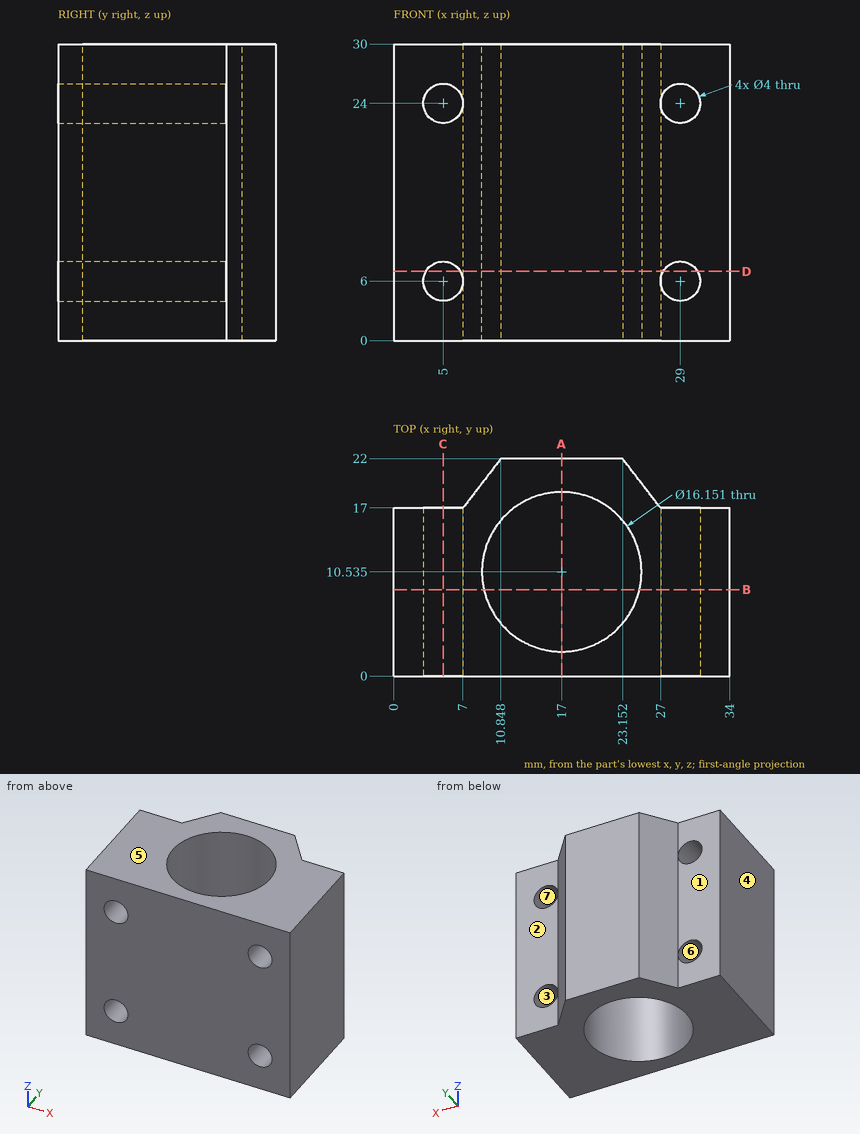
Study the drawing (mm; zero at the part's minimum x, y, z) and answer. A direction names the side the tool comes from. Give positions to 0.01 mm unless a question says otherwise; leave off trailing zeros. Write each loop counter-clockwise with the first axis right and the second up, starting at its lowest first coordinate (ties: lowest second). Pieces come first, ordered by that corner, then holes. Notation, with made-up numbers: (71.25, -32.75) - (75.25, -32.75) arc R24 cw to (75.25, -19.75) - close; hole circle Ø5 at (-3.75, 3). An arc over 180 degrees is marked (long way). One line per question, with ' | ' between items. Start each with the question number.
1. Section D-D, the plane z = 7 is taken. Count the separate pieces of the cut face and the enclosed holes in it, then the cut area to 3 significant figures.
2. Section A-A, the plane x = 17 is taken. Determine the outline of the cut face in (y, z).
3. Section B-B, the plane y = 8.75 is taken. Determine the outline of the cut face in (x, z).
4. Given P1, Ø3.5, axis at x = 31.5, z = 20, coming from the +Y side; P2, Ø10, axis at x = 28.5, z = 20.5, coming from the +Y side; P3, Ø4.5, axis at x = 29, z = 24, coming from the +Y side (1 decimal), each flat-ended and moving along its own axis, determine where each tip first touches the part or whether it passes through.
5. Section C-C, the plane x = 5 is taken. Determine the outline of the cut face in (y, z).
6. For the marked faces 1, 2 and 3, determine the directions among +Z, -Z, +X, -X, +Y, -Y from which every point of the face is accessible in a straight line to the end or side of a thin tool.
7. Straight lines are drawn through the part: line 1 (Z direction, x = 5, y = 7.75); line 2 (X direction, y = 10.5, z = 9.5) (1 decimal); line 3 (X direction, y = 5.5, z = 6) (1 decimal). For each, find the intervals that lie inside material, in ascending order.
8. Determine the mould class of the marked faces 4, 5, 6 and 7 for opening direction Z: +Z half, -Z half, draft (parallel to the pull), parting line (faces both ways), or undercut.
Result:
1) separate pieces: 3 | enclosed holes: 1 | area: 336 mm2
2) outline: (0, 0) - (2.46, 0) - (2.46, 30) - (0, 30) - close; (18.61, 0) - (22, 0) - (22, 30) - (18.61, 30) - close
3) outline: (0, 0) - (9.12, 0) - (9.12, 30) - (0, 30) - close; (24.88, 0) - (34, 0) - (34, 30) - (24.88, 30) - close; hole circle Ø4 at (5, 6); hole circle Ø4 at (5, 24); hole circle Ø4 at (29, 6); hole circle Ø4 at (29, 24)
4) P1: stops at y = 17 | P2: stops at y = 21.55 | P3: stops at y = 17.3
5) outline: (0, 0) - (17, 0) - (17, 4) - (0, 4) - close; (0, 8) - (17, 8) - (17, 22) - (0, 22) - close; (0, 26) - (17, 26) - (17, 30) - (0, 30) - close
6) face 1: +Z, -Z, -X, +Y | face 2: +Z, -Z, +X, +Y | face 3: +Y, -Y
7) line 1: z = 0 to 4, 8 to 22, 26 to 30 | line 2: x = 0 to 8.9, 25.1 to 34 | line 3: x = 0 to 3, 7 to 10.7, 23.3 to 27, 31 to 34
8) face 4: draft | face 5: +Z half | face 6: undercut | face 7: undercut
